```python
from build123d import *

# Parameters (mm, degrees)
SKETCH1_W               = 20
SKETCH1_H               = 100
BOSS_EXTRUDE1_DEPTH     = 5
CUT_EXTRUDE1_DEPTH      = 103.102889283
CUT_EXTRUDE1_DEPTH_BACK = 103.102889283
FILLET1_R               = 2


with BuildPart() as part:
    # Sketch1 → Boss-Extrude1 (new body)
    with BuildSketch(Plane.XY):
        with Locations((10, 50)):
            Rectangle(SKETCH1_W, SKETCH1_H)
    extrude(amount=BOSS_EXTRUDE1_DEPTH)

    # Sketch2 → Cut-Extrude1 (cut, two sides: drawn at the far end of the back side and taken through both)
    with BuildSketch(Plane(origin=(0, 0, 0), x_dir=(1, 0, 0), z_dir=(0, 1, 0)).offset(-CUT_EXTRUDE1_DEPTH_BACK)):
        Polygon((0, 0), (20, -2.4), (20, 0), align=None)
        Polygon((0, -5), (20, -2.6), (20, -5), align=None)
    extrude(amount=CUT_EXTRUDE1_DEPTH + CUT_EXTRUDE1_DEPTH_BACK, mode=Mode.SUBTRACT)

    # Fillet1
    # the kernel refuses this fillet: 2 mm, written as the material it takes off along each edge
    with BuildSketch(Plane(origin=(0, -5.635871325, 0), x_dir=(0, 0, 1), z_dir=(0, 1, 0))) as fillet1_piece_1:
        with BuildLine():
            CenterArc((FILLET1_R * 1.12717426496, FILLET1_R), FILLET1_R, 173.157226587, 96.842773413)
            Line((FILLET1_R * 0.134297426474, FILLET1_R * 1.11914522062), (0, 0))
            Line((0, 0), (FILLET1_R * 1.12717426496, 0))
        make_face()
    extrude(amount=111.27174265, mode=Mode.SUBTRACT)
    with BuildSketch(Plane(origin=(0, -5.635871325, 5), x_dir=(0, 0, -1), z_dir=(0, 1, 0))) as fillet1_piece_2:
        with BuildLine():
            CenterArc((FILLET1_R * 1.12717426496, -FILLET1_R), FILLET1_R, 90, 96.842773413)
            Line((FILLET1_R * 0.134297426474, -FILLET1_R * 1.11914522062), (0, 0))
            Line((0, 0), (FILLET1_R * 1.12717426496, 0))
        make_face()
    extrude(amount=111.27174265, mode=Mode.SUBTRACT)
    with BuildSketch(Plane(origin=(24.964384192, 100, 2.995726103), x_dir=(-0.11914522061843055, 0, 0.9928768384869221), z_dir=(-0.9928768384869221, 0, -0.11914522061843054))) as fillet1_piece_3:
        with BuildLine():
            CenterArc((FILLET1_R, -FILLET1_R), FILLET1_R, 90, 90)
            Line((0, -FILLET1_R), (0, 0))
            Line((0, 0), (FILLET1_R, 0))
        make_face()
    extrude(amount=30.143485299, mode=Mode.SUBTRACT)
    with BuildSketch(Plane(origin=(24.964384192, 100, 2.004273897), x_dir=(-0.11914522061843079, 0, -0.9928768384869221), z_dir=(-0.9928768384869221, 0, 0.11914522061843079))) as fillet1_piece_4:
        with BuildLine():
            CenterArc((FILLET1_R, FILLET1_R), FILLET1_R, 180, 90)
            Line((0, FILLET1_R), (0, 0))
            Line((0, 0), (FILLET1_R, 0))
        make_face()
    extrude(amount=30.143485299, mode=Mode.SUBTRACT)


solid = part.part
```
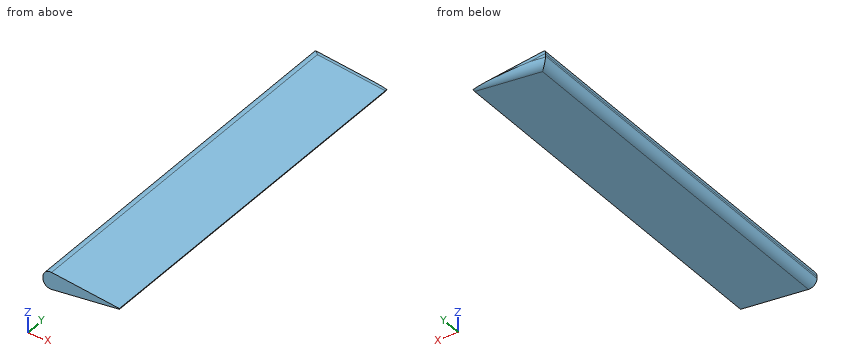
Input: part model. Units: mm. Frame: model coordinates. Coordinates: 2 decimals unless noted, no trailing zeros. Write each loop counter-clockwise with the first axis right and the second up, starting at its lowest first coordinate (ties: lowest second). Pieces come first, ordered by that corner, then holes.
1) Pin query (flat end, axial travel): pin 1 Ø4 at (x, y) = (6, 55) entering from -Z; pin 2 Ø2 at (x, y) = (15, 28) entering from -Z. Return the tip coordinate at first contact, or that it passes through.
2) Material intervals for line 1 along Z through (x, y) = (11.75, 85); line 2 along Z through (x, y) = (14, 94); line 3 along Y through (x, z) = (9, 3.65), sorted ascending.
3) Section A-A on y = 9.5. Output: boundary loops of the cut face in (x, z), and give its area (3 significant figures).
Check result:
1. pin 1: stops at z = 0.48
1. pin 2: stops at z = 1.68
2. line 1: z = 1.41 to 3.59
2. line 2: z = 1.68 to 3.32
2. line 3: y = 0 to 99
3. outline: (0, 2.25) arc R2 ccw to (2.24, 0.27) - (20, 2.4) - (20, 2.6) - (2.24, 4.73) arc R2 ccw to (0, 2.75) - close
3. area: 49.7 mm2
